Part model, mm, in its own coordinate system. Face numbers are marked on the shaded views. A direction names the side the tool comes from. Round coordinates to 2 decimals unless told otherwise and drop trailing zeros. Loops run counter-clockwise (first coordinate to the right, second up) from the corner with the lowest first, then second, coordinate; pieces in that order, holes last. Notation, with made-up numbers: M 75.25,-25.75 L 130.25,-25.75 A12 ccw 130.25,-20.75 Z; hole C 57,14.5 d7. An arc over 180 degrees is marked long. Put each result on its own line as item: value. Start each with the question number.
1) Slice it at B-B on y = 21.5. Give the cut face in (x, z), then the cut area to 3 significant figures.
2) Drop flat-ended pins along their axis: pin 1 Ø8 at (y, z) = (22.5, 2.5) entering from -X; pin 2 Ø1 at (x, y) = (-6, 18) entering from -Z; pin 3 Ø13 at (x, z) = (0, 0) entering from -Y. Give the stop position or say it passes through.
3) Probe line 1 along X through (y, z) = (1.8, 0); line 2 along X through (y, z) = (1.75, -5); line 3 along Y through (x, z) = (-8.5, 11.5). List the from-to ranges inside material, lowest first.
4) Slice it at A-A on y = 12.75. Give the cut face in (x, z) (3 decimals).
5) Which spindle directions (+Z, -Z, +X, -X, +Y, -Y) get a long thin tool onto all of the face, cutting with end or side? Do the marked faces 1, 2, 3, 4 and 5. Say none if no direction does.
6) Pull direction Y, two halves, no side cores. Call the marked faces 6, 7, 8 and 9: +Y half, -Y half, draft (parallel to the pull), parting line (faces both ways), or undercut.
```python
from build123d import *

# Parameters (mm, degrees)
SKETCH5_R         = 4.445
STUB_DEPTH        = 4.104
HEX_2_DEPTH       = 6.985
SKETCH11_W        = 15.24
SKETCH11_H        = 2.54
SKETCH3_R         = 3.302
CENTER_BORE_DEPTH = 36.283163634
FILLET1_R         = 0.254
FILLET2_R         = 0.762
CHAMFER1_SIZE     = 0.508
FILLET3_R         = 0.254


with BuildPart() as part:
    # Sketch1 → Flange (revolve)
    with BuildSketch(Plane(origin=(0, 0, 0), x_dir=(0, 0, -1), z_dir=(1, 0, 0)), mode=Mode.PRIVATE) as flange_sk:
        Polygon((-15, 0), (-15, 3.2), (-7.349295844, 5.25), (0, 5.25), (0, 2.5), (-8.1, 2.5), (-8.1, 0), align=None)
    revolve(flange_sk.sketch.rotate(Axis((0, 0, 0), (0, 1, 0)), 180), axis=Axis((0, 0, 0), (0, 1, 0)))

    # Sketch5 → Stub (add)
    with BuildSketch(Plane.XZ.offset(-2.5)):
        with Locations(Location((0, 0, 0), (0, 0, 270))):
            Circle(SKETCH5_R)
    extrude(amount=-STUB_DEPTH)

    # Sketch6 → Hex 2 (add)
    with BuildSketch(Plane(origin=(0, 6.604, 0), x_dir=(1, 0, 0), z_dir=(0, 1, 0))):
        Polygon((4.106115114, 7.112), (-4.106115114, 7.112), (-8.212230229, 0), (-4.106115114, -7.112), (4.106115114, -7.112), (8.212230229, 0), align=None)
    extrude(amount=HEX_2_DEPTH)

    # Sketch7 → Thread Body (revolve)
    with BuildSketch(Plane.XY, mode=Mode.PRIVATE) as thread_body_sk:
        Polygon((-6.731, 13.589), (-6.274596457, 28.194), (0, 28.194), (0, 13.589), align=None)
    revolve(thread_body_sk.sketch.rotate(Axis((0, 0, 0), (0, 1, 0)), 270), axis=Axis((0, 0, 0), (0, 1, 0)))

    # Sketch11 → Cut-Revolve1 (revolve, cut)
    with BuildSketch(Plane.XY, mode=Mode.PRIVATE) as cut_revolve1_sk:
        with Locations((-14.097, 14.859)):
            Rectangle(SKETCH11_W, SKETCH11_H)
    revolve(cut_revolve1_sk.sketch.rotate(Axis((0, 0, 0), (0, 1, 0)), 270), axis=Axis((0, 0, 0), (0, 1, 0)), mode=Mode.SUBTRACT)

    # Sketch3 → Center Bore (cut, through all)
    with BuildSketch(Plane(origin=(0, 0, 0), x_dir=(1, 0, 0), z_dir=(0, 1, 0))):
        with Locations(Location((0, 0, 0), (0, 0, 270))):
            Circle(SKETCH3_R)
    extrude(amount=CENTER_BORE_DEPTH, mode=Mode.SUBTRACT)

    # Fillet1
    fillet1_edges = [part.edges().sort_by_distance(p)[0] for p in [
        (8.212230229, 10.0965, 0),
        (4.106115114, 10.0965, -7.112),
        (-4.106115114, 10.0965, -7.112),
        (-8.212230229, 10.0965, 0),
        (-4.106115114, 10.0965, 7.112),
        (4.106115114, 10.0965, 7.112),
    ]]
    fillet(fillet1_edges, radius=FILLET1_R)

    # Fillet2
    fillet2_edges = [part.edges().sort_by_distance(p)[0] for p in [
        (0, 3.2, 15),
    ]]
    fillet(fillet2_edges, radius=FILLET2_R)

    # Chamfer1
    chamfer1_edges = [part.edges().sort_by_distance(p)[0] for p in [
        (0, 28.194, -3.302),
    ]]
    chamfer(chamfer1_edges, length=CHAMFER1_SIZE)

    # Fillet3
    fillet3_edges = [part.edges().sort_by_distance(p)[0] for p in [
        (0, 13.589, 6.477),
    ]]
    fillet(fillet3_edges, radius=FILLET3_R)


solid = part.part
```
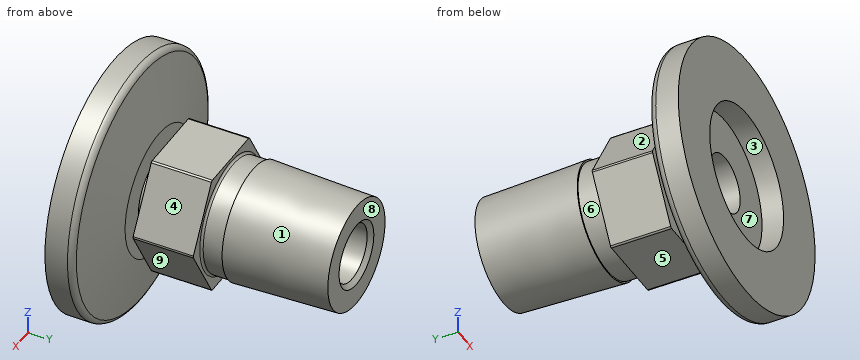
Recorded:
1. outline: C 0,0 d12.97; hole C 0,0 d6.6
1. area: 97.8 mm2
2. pin 1: stops at x = -6.55
2. pin 2: stops at z = -3.64
2. pin 3: stops at y = 2.5
3. line 1: x = -15 to -8.1, 8.1 to 15
3. line 2: x = -14.14 to -6.37, 6.37 to 14.14
3. line 3: y = 0 to 3.39
4. outline: M -8.139,-0.127 L -4.179,-6.985 A0.254 ccw -3.959,-7.112 L 3.959,-7.112 A0.254 ccw 4.179,-6.985 L 8.139,-0.127 A0.254 ccw 8.139,0.127 L 4.179,6.985 A0.254 ccw 3.959,7.112 L -3.959,7.112 A0.254 ccw -4.179,6.985 L -8.139,0.127 A0.254 ccw Z; hole C 0,0 d6.604
5. face 1: +Y
5. face 2: +Z, -X, +Y
5. face 3: -Y
5. face 4: +Z, +X, +Y
5. face 5: -Z, +X, -X, +Y
6. face 6: undercut
6. face 7: -Y half
6. face 8: +Y half
6. face 9: draft
